```python
from build123d import *

# Parameters (mm, degrees)
BOSS_EXTRUDE1_DEPTH      = 5
BOSS_EXTRUDE1_DEPTH_BACK = 5
SKETCH3_W                = 38
SKETCH3_H                = 26
BOSS_EXTRUDE2_DEPTH      = 3
M3_CLEARANCE_HOLE1_D     = 3.4
M3_CLEARANCE_HOLE1_DEPTH = 3
FILLET3_R                = 2
M3_CLEARANCE_HOLE2_D     = 3.4
M3_CLEARANCE_HOLE2_DEPTH = 10
M3_CLEARANCE_HOLE2_TIP   = 1.021463052
SKETCH4_W                = 28
SKETCH4_H                = 12.861112754
CUT_EXTRUDE2_DEPTH       = 3


with BuildPart() as part:
    # Sketch1 → Boss-Extrude1 (new, two sides: drawn at the far end of the back side and taken through both)
    with BuildSketch(Plane.XY.offset(-BOSS_EXTRUDE1_DEPTH_BACK)):
        Polygon((19, -3), (-19, -3), (-19, 44.583333333), (-19, 79.5), (-10.5, 79.5), (-10.5, 76.5), (-16, 76.5), (-16, 0), (16, 0), (16, 76.5), (10.5, 76.5), (10.5, 79.5), (19, 79.5), align=None)
    extrude(amount=BOSS_EXTRUDE1_DEPTH + BOSS_EXTRUDE1_DEPTH_BACK)

    # Sketch3 → Boss-Extrude2 (add)
    with BuildSketch(Plane(origin=(0, -3, 0), x_dir=(-1, 0, 0), z_dir=(0, -1, 0))):
        Rectangle(SKETCH3_W, SKETCH3_H)
    extrude(amount=-BOSS_EXTRUDE2_DEPTH)

    # M3 Clearance Hole1
    with Locations(Plane(origin=(0, 79.5, 0), x_dir=(1, 0, 0), z_dir=(0, 1, 0))):
        with Locations((-13, 0), (13, 0)):
            Hole(M3_CLEARANCE_HOLE1_D / 2, depth=M3_CLEARANCE_HOLE1_DEPTH)

    # Fillet3
    fillet3_edges = [part.edges().sort_by_distance(p)[0] for p in [
        (-16, 0, 0),
        (16, 0, 0),
    ]]
    fillet(fillet3_edges, radius=FILLET3_R)

    # M3 Clearance Hole2
    with Locations(Plane(origin=(0, 0, 0), x_dir=(1, 0, 0), z_dir=(0, 1, 0))):
        with Locations((16.679968376, -8), (-16.340858472, -8), (16.679968376, 8), (-16.340858472, 8)):
            Hole(M3_CLEARANCE_HOLE2_D / 2, depth=M3_CLEARANCE_HOLE2_DEPTH)
            with Locations((0, 0, -(M3_CLEARANCE_HOLE2_DEPTH + M3_CLEARANCE_HOLE2_TIP / 2))):  # 118° drill point
                Cone(0, M3_CLEARANCE_HOLE2_D / 2, M3_CLEARANCE_HOLE2_TIP, mode=Mode.SUBTRACT)

    # Sketch4 → Cut-Extrude2 (cut)
    with BuildSketch(Plane.XZ.offset(3)):
        Rectangle(SKETCH4_W, SKETCH4_H)
    extrude(amount=-CUT_EXTRUDE2_DEPTH, mode=Mode.SUBTRACT)


solid = part.part
```
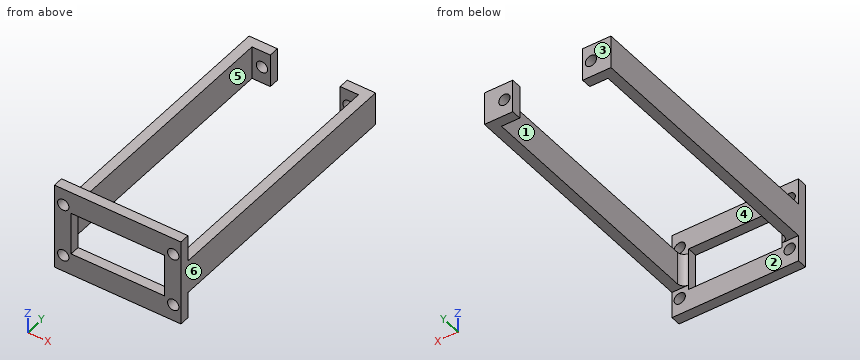
Geometry: final body of the model. Coordinates: model frame, mm. Face numbers are marked on the shaded views. A direction names the side the tool comes from. Coordinates: 2 decimals unless noted, no trailing zeros. Order: outer loops, then holes, each group sorted by start corner. A loop starts at its lowest first (then second) coordinate and runs counter-clockwise, first axis right, second up. Notation, with made-up numbers: M -39,-4.5 L 14,-4.5 A8 cw 14,0.5 Z; hole C 23,0 d10. An arc over 180 degrees is marked long. Answer in a Markdown table with one row per item. Add a question column.
Q1. Reachability of the marked faces 1, 2 and 3 from +Z, -Z, +X, -X, +Y, -Y: full face, straight path, thin tool, end or side. Return the list, or none.
Q2. Contact query for flat-ended pins moving along their axis: P1, Ø4, axis at x = -15, y = 53.5, coming from the -Z side; P2, Ø10, axis at y = 21.5, z = -6.5, coming from the +X side; P3, Ø9, axis at x = -4, z = 7.5, coming from the +Y side. Output: stop coordinate, or through.
Q3. Section query A-A on y = 46.5. Return the cut outline in (x, z).
Q4. Mould query, pull axis X, two halves, no side actions, for the marked faces 4, 5 and 6. Classes: released by +X, released by -X, zero draft, split by the parting line, or undercut.
Q5. Section query B-B on x = -13. Return the cut outline in (y, z), and give its area (3 significant figures).
Q6. Section query C-C on z = -8. Return the cut outline in (x, y), and give its area (3 significant figures).
Q7. Section query D-D on z = 0. Return the cut outline in (x, y).
Q8. Line query: L1, parallel to X at y = -0.8, z = -8; L2, parallel to X at y = 29, z = 2.75; L3, parallel to Z at x = 13, y = 77.2. Output: solid intervals per line, ascending.
Completed:
| question | item | result |
|---|---|---|
| 1 | face 1 | +Z, -Z |
| 1 | face 2 | -Z, +X, -X, +Y |
| 1 | face 3 | +Z, -Z, +X, -X, +Y |
| 2 | P1 | stops at z = -5 |
| 2 | P2 | stops at x = 19 |
| 2 | P3 | stops at y = 0 |
| 3 | outline | M -19,-5 L -16,-5 L -16,5 L -19,5 Z; M 16,-5 L 19,-5 L 19,5 L 16,5 Z |
| 4 | face 4 | zero draft |
| 4 | face 5 | undercut |
| 4 | face 6 | released by +X |
| 5 | outline | M -3,-13 L 0,-13 L 0,-6.43 L -3,-6.43 Z; M -3,6.43 L 0,6.43 L 0,13 L -3,13 Z; M 76.5,-5 L 79.5,-5 L 79.5,-1.7 L 76.5,-1.7 Z; M 76.5,1.7 L 79.5,1.7 L 79.5,5 L 76.5,5 Z |
| 5 | area | 59.2 mm2 |
| 6 | outline | M -19,-3 L -18.04,-3 L -18.04,0 L -19,0 Z; M -14.64,-3 L 14.98,-3 L 14.98,0 L -14.64,0 Z; M 18.38,-3 L 19,-3 L 19,0 L 18.38,0 Z |
| 6 | area | 93.6 mm2 |
| 7 | outline | M -19,-3 L -14,-3 L -14,0 A2 cw -16,2 L -16,76.5 L -14.7,76.5 L -14.7,79.5 L -19,79.5 Z; M -11.3,76.5 L -10.5,76.5 L -10.5,79.5 L -11.3,79.5 Z; M 10.5,76.5 L 11.3,76.5 L 11.3,79.5 L 10.5,79.5 Z; M 14,-3 L 19,-3 L 19,79.5 L 14.7,79.5 L 14.7,76.5 L 16,76.5 L 16,2 A2 cw 14,0 Z |
| 8 | L1 | x = -19 to -18.04, -14.64 to 14.98, 18.38 to 19 |
| 8 | L2 | x = -19 to -16, 16 to 19 |
| 8 | L3 | z = -5 to -1.7, 1.7 to 5 |
